Source: three-view drawing plus pictorial views. Frame: mm from the lowest corner of the part. A direction names the side the tool comes from. Coordinates: 2 decimals unless noted, no trailing zeros. Loops run counter-clockwise (first coordinate to the right, second up) from the corner with the lowest first, then second, coordinate; pieces in that order, holes last. Notation, with made-up numbers: (72.25, -14.5) - (81.25, -14.5) arc R15 cw to (81.25, 10.5) - close; hole circle Ø9 at (10, 41). An arc over 180 degrees is marked (long way). Use CSV: the item, a comma, the result in double quotes. Start each with the question number.
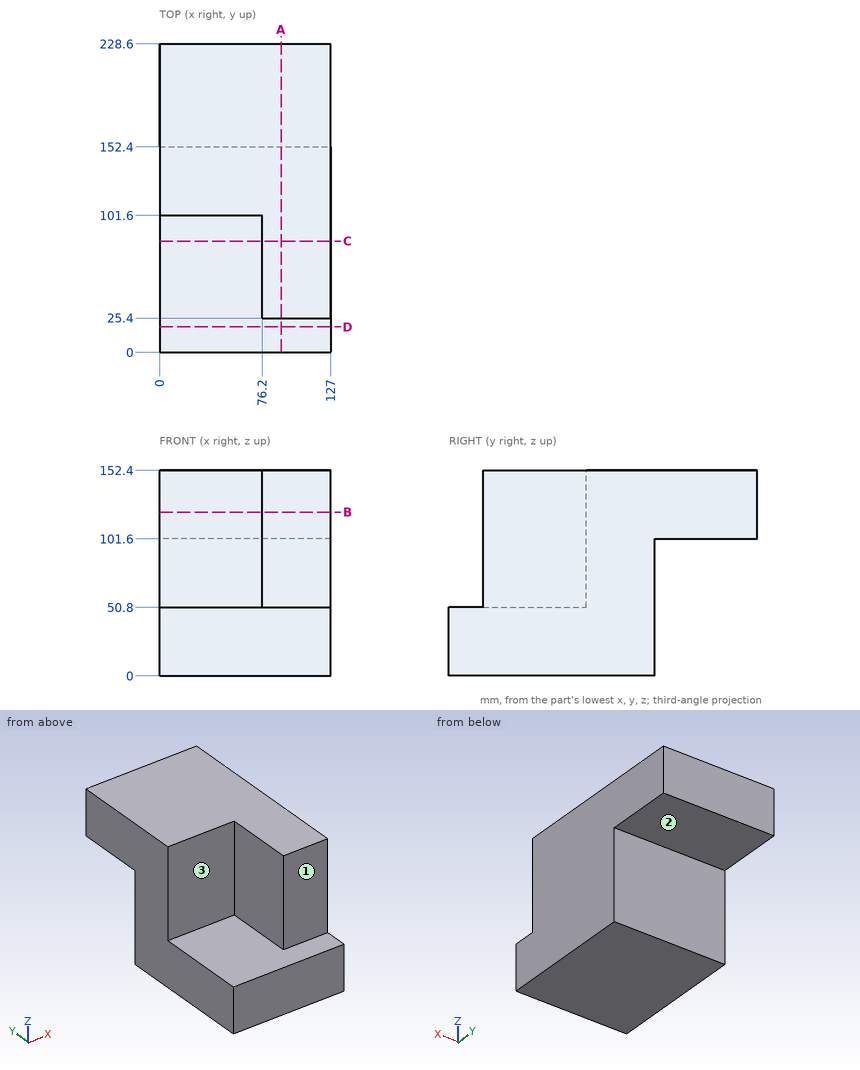
(1) Section C-C on y = 82.5. Output: boundary loops of the cut face in (x, z), plus the area to 3 significant figures.
(2) Ray query, line 1 (Y direction, x = 42.5, z = 77); line 2 (Y direction, x = 83.5, z = 46); line 3 (X direction, y = 48.5, z = 87). Return the intervals inside material, ascending. Write a range as [from, to].
(3) Section D-D on y = 19. Output: boundary loops of the cut face in (x, z), plus the area to 3 significant figures.
(4) Reachability of the marked faces 1, 2 and 3 from +Z, -Z, +X, -X, +Y, -Y: full face, straight path, thin tool, end or side. Return the list, or none.
(5) Section A-A on x = 90. Output: boundary loops of the cut face in (y, z), plus the area to 3 significant figures.
(6) Pin query (flat end, axial travel): pin 1 Ø1 at (x, z) = (20, 93) entering from -Y; pin 2 Ø12 at (y, z) = (90.5, 31.5) entering from -X. Return the tip coordinate at first contact, or that it passes through.
(7) Section B-B on z = 121.5. Output: boundary loops of the cut face in (x, y), plus the area to 3 significant figures.
Solution:
1,outline,"(0, 0) - (127, 0) - (127, 152.4) - (76.2, 152.4) - (76.2, 50.8) - (0, 50.8) - close"
1,area,"11,600 mm²"
2,line 1,"y = [101.6, 152.4]"
2,line 2,"y = [0, 152.4]"
2,line 3,"x = [76.2, 127]"
3,outline,"(0, 0) - (127, 0) - (127, 50.8) - (0, 50.8) - close"
3,area,"6,450 mm²"
4,face 1,"+Z, +X, -X, -Y"
4,face 2,"-Z, +X, -X, +Y"
4,face 3,"+Z, -X, -Y"
5,outline,"(0, 0) - (152.4, 0) - (152.4, 101.6) - (228.6, 101.6) - (228.6, 152.4) - (25.4, 152.4) - (25.4, 50.8) - (0, 50.8) - close"
5,area,"24,500 mm²"
6,pin 1,"stops at y = 101.6"
6,pin 2,"stops at x = 0"
7,outline,"(0, 101.6) - (76.2, 101.6) - (76.2, 25.4) - (127, 25.4) - (127, 228.6) - (0, 228.6) - close"
7,area,"20,000 mm²"
